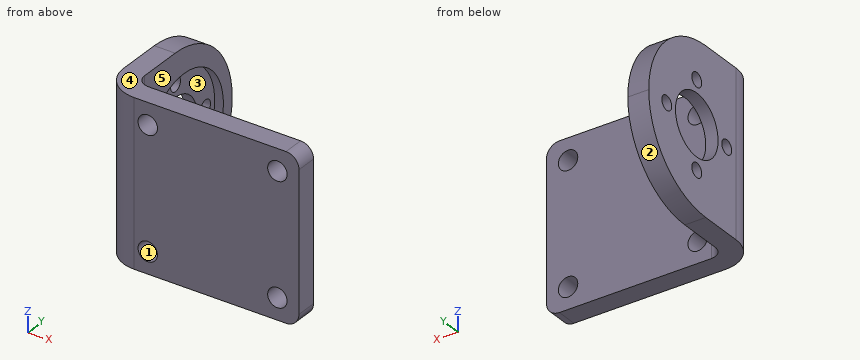
from build123d import *

# Parameters (mm, degrees)
T_LE_DE_BASE_PLI_E1_DEPTH    = 38
ENL_V_MAT_EXTRU_1_DEPTH      = 68.129147917
ENL_V_MAT_EXTRU_1_DEPTH_BACK = 68.129147917
ESQUISSE6_R                  = 7.1
ESQUISSE7_R                  = 13.05
ENL_V_MAT_EXTRU_2_DEPTH      = 2
CONG_1_R                     = 19
ENL_V_MAT_EXTRU_3_DEPTH      = 69.373404917
ENL_V_MAT_EXTRU_3_DEPTH_BACK = 69.373404917
ESQUISSE8_R                  = 1.65
ENL_V_MAT_EXTRU_4_DEPTH      = 68.77626797
ENL_V_MAT_EXTRU_4_DEPTH_BACK = 68.77626797
ESQUISSE9_R                  = 2.25
CONG_2_R                     = 3


# Read off the part's stored shape, not the designer's step: Tôle de base pliée1
with BuildPart() as part:
    # Tôle de base pliée1 outline → Tôle de base pliée1 (new body)
    with BuildSketch(Plane.XY):
        with BuildLine():
            Line((4.85, 7.85), (4.85, 37))
            Line((4.85, 37), (0, 37))
            Line((0, 37), (0, 7.85))
            ThreePointArc((0, 7.85), (2.299211768, 2.299211768), (7.85, 0))
            Line((7.85, 0), (46, 0))
            Line((46, 0), (46, 4.85))
            Line((46, 4.85), (7.85, 4.85))
            ThreePointArc((7.85, 4.85), (5.728679656, 5.728679656), (4.85, 7.85))
        make_face()
    extrude(amount=T_LE_DE_BASE_PLI_E1_DEPTH)

    # Esquisse6 → Enlèv. mat.-Extru.1 (cut, two sides: drawn at the far end of the back side and taken through both)
    with BuildSketch(Plane(origin=(4.85, 0, 0), x_dir=(0, 0, -1), z_dir=(1, 0, 0)).offset(-ENL_V_MAT_EXTRU_1_DEPTH_BACK)):
        with Locations((-19, 21)):
            Circle(ESQUISSE6_R)
    extrude(amount=ENL_V_MAT_EXTRU_1_DEPTH + ENL_V_MAT_EXTRU_1_DEPTH_BACK, mode=Mode.SUBTRACT)

    # Esquisse7 → Enlèv. mat.-Extru.2 (cut)
    with BuildSketch(Plane(origin=(4.85, 0, 0), x_dir=(0, 0, -1), z_dir=(1, 0, 0))):
        with Locations((-19, 21)):
            Circle(ESQUISSE7_R)
    extrude(amount=-ENL_V_MAT_EXTRU_2_DEPTH, mode=Mode.SUBTRACT)

    # Congé1
    cong_1_edges = [part.edges().sort_by_distance(p)[0] for p in [
        (2.425, 37, 0),
        (2.425, 37, 38),
    ]]
    fillet(cong_1_edges, radius=CONG_1_R - 0.0001)  # a hair under: the kernel refuses the full size

    # Esquisse8 → Enlèv. mat.-Extru.3 (cut, two sides: drawn at the far end of the back side and taken through both)
    with BuildSketch(Plane(origin=(2.85, 0, 0), x_dir=(0, 0, -1), z_dir=(1, 0, 0)).offset(-ENL_V_MAT_EXTRU_3_DEPTH_BACK)):
        with Locations((-9, 21)):
            Circle(ESQUISSE8_R)
        with Locations((-19, 11)):
            Circle(ESQUISSE8_R)
        with Locations((-29, 21)):
            Circle(ESQUISSE8_R)
        with Locations((-19, 31)):
            Circle(ESQUISSE8_R)
    extrude(amount=ENL_V_MAT_EXTRU_3_DEPTH + ENL_V_MAT_EXTRU_3_DEPTH_BACK, mode=Mode.SUBTRACT)

    # Esquisse9 → Enlèv. mat.-Extru.4 (cut, two sides: drawn at the far end of the back side and taken through both)
    with BuildSketch(Plane(origin=(0, 4.85, 0), x_dir=(1, 0, 0), z_dir=(0, 1, 0)).offset(-ENL_V_MAT_EXTRU_4_DEPTH_BACK)):
        with Locations(Location((41, -5, 0), (0, 0, 270))):
            Circle(ESQUISSE9_R)
        with Locations(Location((11, -5, 0), (0, 0, 90))):
            Circle(ESQUISSE9_R)
        with Locations(Location((11, -33, 0), (0, 0, 270))):
            Circle(ESQUISSE9_R)
        with Locations(Location((41, -33, 0), (0, 0, 90))):
            Circle(ESQUISSE9_R)
    extrude(amount=ENL_V_MAT_EXTRU_4_DEPTH + ENL_V_MAT_EXTRU_4_DEPTH_BACK, mode=Mode.SUBTRACT)

    # Congé2
    cong_2_edges = [part.edges().sort_by_distance(p)[0] for p in [
        (46, 2.425, 38),
        (46, 2.425, 0),
    ]]
    fillet(cong_2_edges, radius=CONG_2_R)


solid = part.part
The listing builds one solid part. Answer for the finished solid, in the listing's coordinates (mm). Face numbers are marked on the shaded views. A direction names the side the tool comes from. Round coordinates to 2 decimals unless told otherwise and drop trailing zeros. Order: outer loops, then holes, each group sorted by start corner. A loop starts at its lowest first (then second) coordinate and runs counter-clockwise, first axis right, second up. Notation, with made-up numbers: (39, 83) -> (98, 83) arc R22 ccw to (98, 113) -> close; hole circle Ø3 at (11.5, -3). An arc over 180 degrees is marked (long way). Write each question's results on one line, items separated by ' | '. Start each with the question number.
Q1. The mould has two halves that part along X. Classify the marked faces 1, 2 and 3: pulls with the +X half, pulls with the -X half, needs draft (parallel to the pull), parting line crosses it, or undercut.
Q2. Each of these flat-tipped pins is pushed along its axis until it touches: pin 1 (19 mm diameter, centred on x = 24.5, z = 13.5, fed in from +Y); pin 2 (2.5 mm diameter, centred on x = 41, z = 33, fed in from -Y); pin 3 (21 mm diameter, centred on y = 24.5, z = 20.5, fed in from +X); pin 4 (4 mm diameter, centred on x = 6.5, y = 27, fed in from -Z). Where does it stop, or does it pass through?
Q3. Straight lines are drawn through the part: probe 1 along Z at (x, y) = (1.75, 21); probe 2 along X at (y, z) = (12, 5); probe 3 along Y at (x, z) = (2.2, 19). For each, find the intervals that lie inside material, in ascending order. Write a range as from..to.
Q4. Find section C-C (z = 33.5). Determine the outline of the cut face in (x, y).
Q5. Find section D-D (z = 29). Determine the outline of the cut face in (x, y), then the cut area to 3 significant figures.
Q6. Find section A-A (x = 11). Determine the outline of the cut face in (y, z).
Q7. Find section B-B (y = 31). Determine the outline of the cut face in (x, z).
Q8. Which of the six approach directions +Z, -Z, +X, -X, +Y, -Y give full straight-line access (tool end or side, diameter ignored) to the marked faces 4 and 5?
Worked answers:
1) face 1: undercut | face 2: needs draft | face 3: pulls with the +X half
2) pin 1: stops at y = 4.85 | pin 2: passes through | pin 3: stops at x = 4.85 | pin 4: stops at z = 1.71
3) probe 1: z = 0.24..7.35, 10.65..11.9, 26.1..27.35, 30.65..37.76 | probe 2: x = 0..4.85 | probe 3: y = 2.4..9.35, 12.65..13.9, 28.1..29.35, 32.65..37
4) outline: (0, 7.85) arc R7.85 ccw to (7.85, 0) -> (8.81, 0) -> (8.81, 4.85) -> (7.85, 4.85) arc R3 cw to (4.85, 7.85) -> (4.85, 30.28) -> (0, 30.28) -> close; (13.19, 0) -> (38.81, 0) -> (38.81, 4.85) -> (13.19, 4.85) -> close; (43.19, 0) -> (46, 0) -> (46, 4.85) -> (43.19, 4.85) -> close
5) outline: (0, 7.85) arc R7.85 ccw to (7.85, 0) -> (46, 0) -> (46, 4.85) -> (7.85, 4.85) arc R3 cw to (4.85, 7.85) -> (4.85, 12.62) -> (2.85, 12.62) -> (2.85, 19.35) -> (0, 19.35) -> close; (0, 22.65) -> (2.85, 22.65) -> (2.85, 29.38) -> (4.85, 29.38) -> (4.85, 34.16) -> (0, 34.16) -> close | area: 311 mm2
6) outline: (0, 0) -> (4.85, 0) -> (4.85, 2.75) -> (0, 2.75) -> close; (0, 7.25) -> (4.85, 7.25) -> (4.85, 30.75) -> (0, 30.75) -> close; (0, 35.25) -> (4.85, 35.25) -> (4.85, 38) -> (0, 38) -> close
7) outline: (0, 5.14) -> (4.85, 5.14) -> (4.85, 10.62) -> (2.85, 10.62) -> (2.85, 17.35) -> (0, 17.35) -> close; (0, 20.65) -> (2.85, 20.65) -> (2.85, 27.38) -> (4.85, 27.38) -> (4.85, 32.86) -> (0, 32.86) -> close
8) face 4: +Z, +X, -X, +Y, -Y | face 5: +Z, -Z, +X, +Y
